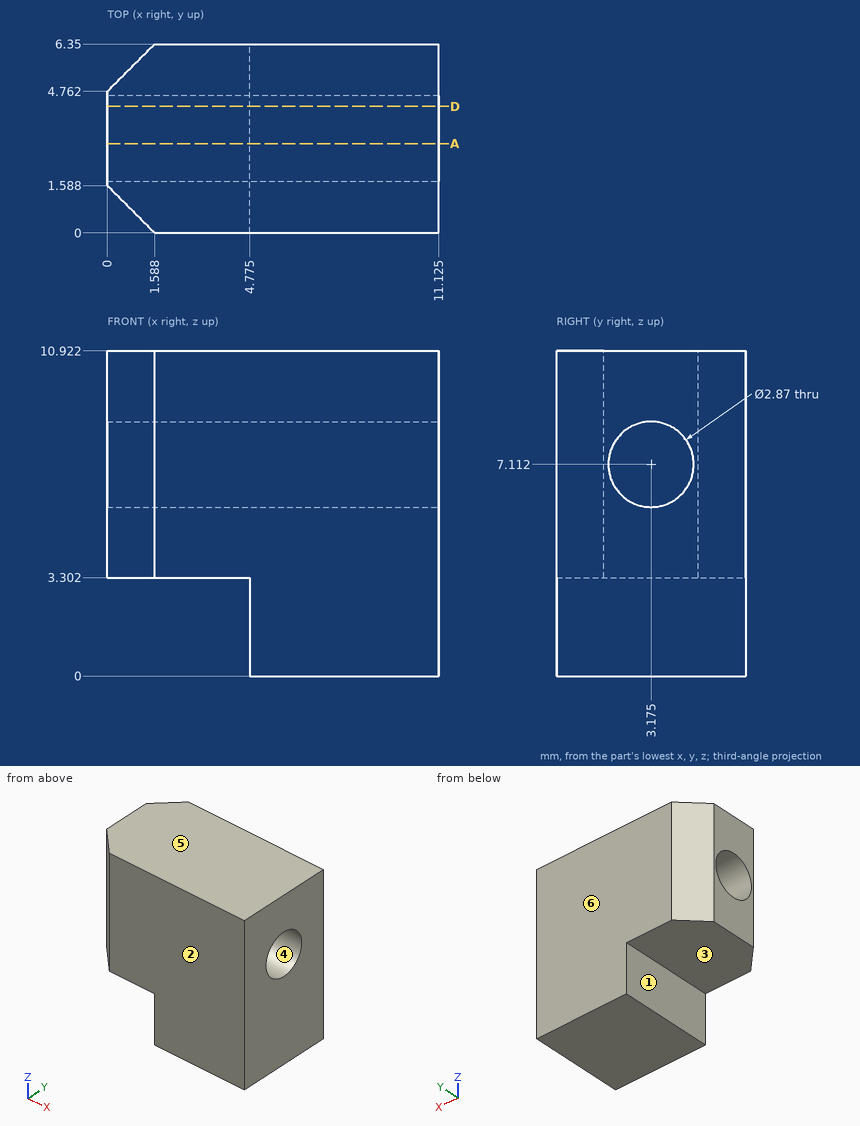
Geometry: see drawing. Coordinates: mm, zero at the bounding-box minimum. A direction names the side the tool comes from. Round coordinates to 2 decimals unless told otherwise and drop trailing zeros. Write each loop counter-clockwise with the first axis right and the second up, starting at its lowest first coordinate (ties: lowest second). Pieces come first, ordered by that corner, then holes.
Item 1: Set-up query: the marked faces 1 and 2. Return all of +Z, -Z, +X, -X, +Y, -Y with unobstructed straight access to the full face (end or side cutting, diameter ignored); none if empty.
Item 2: Section query A-A (y = 3). Return loops of the section in (x, z) (1 decimal).
Item 3: Section query D-D (y = 4.25). Return loops of the section in (x, z) (1 decimal).
Item 4: Material intervals for L1, parallel to Z at x = 4, y = 2.75; L2, parallel to Y at x = 8, z = 7.75; L3, parallel to Z at x = 8, y = 3.75 (1 decimal), sorted ascending.
Item 5: Pin query (flat end, axial travel): P1, Ø3.5, axis at y = 3.5, z = 2, coming from the -X side; P2, Ø2.5, axis at x = 3, y = 2, coming from the -Z side; P3, Ø2, axis at y = 0.5, z = 2, coming from the -X side (1 decimal). Return the tip coordinate at first contact, or that it passes through.
Item 6: Mould query, pull axis Z, two halves, no side actions, for the marked faces 3, 4, 5 and 6. Classes: +Z half, -Z half, draft (parallel to the pull), parting line (faces both ways), or undercut.
Completed:
1. face 1: -Z, -X, +Y, -Y
1. face 2: +Z, -Z, +X, -X, -Y
2. outline: (0, 3.3) - (4.8, 3.3) - (4.8, 0) - (11.1, 0) - (11.1, 5.7) - (0, 5.7) - close; (0, 8.5) - (11.1, 8.5) - (11.1, 10.9) - (0, 10.9) - close
3. outline: (0, 3.3) - (4.8, 3.3) - (4.8, 0) - (11.1, 0) - (11.1, 6.2) - (0, 6.2) - close; (0, 8.1) - (11.1, 8.1) - (11.1, 10.9) - (0, 10.9) - close
4. L1: z = 3.3 to 5.74, 8.48 to 10.92
4. L2: y = 0 to 1.89, 4.46 to 6.35
4. L3: z = 0 to 5.8, 8.4 to 10.9
5. P1: stops at x = 0
5. P2: stops at z = 3.3
5. P3: stops at x = 4.8
6. face 3: -Z half
6. face 4: undercut
6. face 5: +Z half
6. face 6: draft
